Verification items for the finished model (mm, model axes). Face numbers are marked on the shaded views. A direction names the side the tool comes from. Round coordinates to 2 decimals unless told otherwise and drop trailing zeros. Order: outer loops, then holes, each group sorted by start corner. A loop starts at its lowest first (then second) coordinate and runs counter-clockwise, first axis right, second up. Notation, with made-up numbers: M -30.5,23.5 L -7.5,23.5 A21 cw -7.5,33.5 Z; hole C -31,35 d4. An arc over 180 degrees is marked long. Use CSV: the item, a comma, the result in double quotes. Start each with the question number.
Q1. Gauge pin test, flat ends, axial feed: pin 1 Ø1.2 at (x, z) = (-4, -0.5) entering from +Y; pin 2 Ø3.5 at (y, z) = (6.5, 1.5) entering from +X; pin 3 Ø1 at (x, z) = (22, 1.5) entering from -Y; pin 4 Ø1.5 at (x, y) = (13, 7.5) entering from -Z. Record the tip position at first contact, or that the pin passes through.
Q2. Set-up check for the marked faces 5 and 6: record each of +Z, -Z, +X, -X, +Y, -Y from which the full face is reachable in a straight line by a thin tool's end or side.
Q3. Sectioned sample at C-C (x = 23). Enter the section's corners in (y, z), and give its area (3 significant figures).
Q4. Sectioned sample at D-D (x = 0). Enter the section's corners in (y, z), and give its area (3 significant figures).
Q5. Scan lines: line 1 (Y direction, x = -8.5, z = 0); line 2 (X direction, y = 7.5, z = 2); line 3 (Y direction, x = 4.5, z = -0.25). Record each from-to range of solid material in increasing order.
Q6. Sectioned sample at A-A (y = 7.75). Enter the section's corners in (x, z), and give its area (3 significant figures).
Q7. Mould release check, pull along X, two halves, no side actions. Record for the marked faces 1, 2, 3 and 4: +X half, -X half, draft (parallel to the pull), parting line (faces both ways), or undercut.
Q8. Sectioned sample at B-B (z = 2.5). Enter the section's corners in (x, y).
Autodesk Inventor part; units mm, degrees
ref_plane "Arbeitsebene1" through (0.8295, 8.6008, 0) normal (0, 1, 0) x (-1, 0, 0)
ref_plane "Arbeitsebene2" through (-6.6705, 4.6008, 0) normal (-1, 0, 0) x (0, 0, 1)
ref_plane "YZ Ebene" through (0, 0, 0) normal (1, 0, 0) x (0, 1, 0)
sketch "Skizze1" plane through (0, 0, 0) normal (0, 0, 1) x (1, 0, 0)
  line L0 (-16.1705, 4.6008) -> (-16.1705, 8.6008)
  line L1 (-16.1705, 8.6008) -> (17.8295, 8.6008)
  line L2 (17.8295, 8.6008) -> (17.8295, 6.6008)
  line L3 (17.8295, 6.6008) -> (29.8295, 6.6008)
  line L4 (29.8295, 6.6008) -> (29.8295, 4.6008)
  line L5 (29.8295, 4.6008) -> (-16.1705, 4.6008)
  dimension "d0" = 46
  dimension "d1" = 12
  dimension "d2" = 4
  dimension "d3" = 8
revolve "Grundkörper" add sketch "Skizze1" angle 360 about axis through (29.8295, 4.6008, 0) along (-1, 0, 0)
sketch "Skizze2" plane through (-16.1705, 4.6008, 0) normal (-1, 0, 0) x (0, 0, 1)
  circle A0 centre (0, 0) radius 4
hole "3,2 Bohrung axial" at (-16.1705, 4.6008, 0) direction (1, 0, 0) diameter 3.2 depth 14 tip angle 118
chamfer "Fase 0,5x45" distance 0.5 angle 45 1 edges at (29.8295, 2.6008, 0)
ref_plane "Arbeitsebene1" through (0.8295, 8.6008, 0) normal (0, 1, 0) x (-1, 0, 0)
sketch "Skizze3" plane through (0.8295, 8.6008, 0) normal (0, 1, 0) x (-1, 0, 0)
  line L0 (17, 4) -> (17, -4)
  point P0 (5.5, 0)
  dimension "d14" = 11.5
hole "3,2 Bohrung radial" at (-4.6705, 8.6008, 0) direction (0, -1, 0) diameter 3.2 end up to surface
ref_plane "Arbeitsebene2" through (-6.6705, 4.6008, 0) normal (-1, 0, 0) x (0, 0, 1)
sketch "Skizze5" plane through (-6.6705, 4.6008, 0) normal (-1, 0, 0) x (0, 0, 1)
  line L0 (-1.6, 0) -> (-1.6, 3.6661)
  circle A0 centre (0, 0) radius 4
  line L1 (1.6, 0) -> (1.6, 3.6661)
  line L2 (-3.9383, 0.7) -> (-2.1, 2.5)
  line L3 (-2.1, 2.5) -> (2.1, 2.5)
  line L4 (2.1, 2.5) -> (3.7081, 1.5)
  line L5 (3.1225, -2.5) -> (-3.1225, -2.5)
  line L6 (0, -4) -> (0, 4) construction
  dimension "d31" = 1.5
  dimension "d32" = 4
  dimension "d33" = 3.2
  dimension "d34" = 5
  dimension "d35" = 0.5
  dimension "d36" = 0.5
extrude "Entlüftungssteuerschlitz" cut sketch "Skizze5" against normal blind 4 contours L3 L2 A0 L0 | L0 A0 L1 L3 | L1 A0 L4 L3
extrude "Belüftungssteuerschlitz" cut sketch "Skizze5" against normal blind 12 contours L5 A0
properties part number "Kurbelwelle" material "CuZn40"
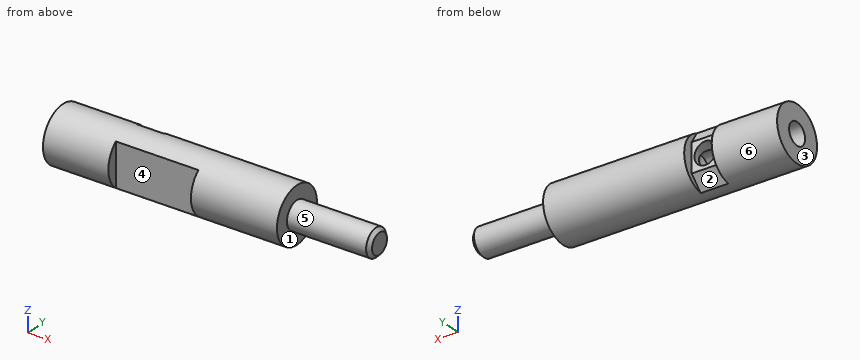
Verdict:
1,pin 1,"stops at y = 3.44"
1,pin 2,"stops at x = 29.83"
1,pin 3,"stops at y = 2.87"
1,pin 4,"stops at z = -3.37"
2,face 5,"+X"
2,face 6,"+X, -X"
3,outline,"C 4.6,0 d4"
3,area,"12.6 mm²"
4,outline,"M 2.1,-3.12 A4 ccw long 2.1,3.12 Z"
4,area,"43.7 mm²"
5,line 1,"y = 0.6 to 3, 6.2 to 8.6"
5,line 2,"x = -16.17 to -6.67, -2.67 to 17.83"
5,line 3,"y = 2.1 to 8.59"
6,outline,"M -16.17,-2.47 L -6.67,-2.47 L -6.67,2.47 L -16.17,2.47 Z; M -2.67,-2.47 L 17.83,-2.47 L 17.83,2.47 L -2.67,2.47 Z"
6,area,"148 mm²"
7,face 1,"+X half"
7,face 2,"undercut"
7,face 3,"-X half"
7,face 4,"undercut"
8,outline,"M -16.17,1.48 L -6.67,1.48 L -6.67,2.1 L 5.33,2.1 L 5.33,1.48 L 17.83,1.48 L 17.83,7.72 L -2.67,7.72 L -2.67,6.85 L -6.67,6.85 L -6.67,7.72 L -16.17,7.72 Z"
